```python
from build123d import *

# Parameters (mm, degrees)
SKETCH_1_W          = 120
SKETCH_1_H          = 170
SKETCH_1_R          = 1.7
EXTRUDE_1_DEPTH     = 7
SKETCH_3_R          = 3.4
CUT_EXTRUDE_1_DEPTH = 3
FILLET_1_R          = 5


with BuildPart() as part:
    # 草图1 → 凸台-拉伸1 (new body)
    with BuildSketch(Plane(origin=(0, 0, 0), x_dir=(1, 0, 0), z_dir=(0, 1, 0))):
        with Locations((4.775862069, 0)):
            Rectangle(SKETCH_1_W, SKETCH_1_H)
        with Locations((-8.724137931, 16.5)):
            Circle(SKETCH_1_R, mode=Mode.SUBTRACT)
        with Locations((18.275862069, 16.5)):
            Circle(SKETCH_1_R, mode=Mode.SUBTRACT)
        with Locations((18.275862069, -16.5)):
            Circle(SKETCH_1_R, mode=Mode.SUBTRACT)
        with Locations((-8.724137931, -16.5)):
            Circle(SKETCH_1_R, mode=Mode.SUBTRACT)
        with Locations((-2.724137931, 3)):
            Circle(SKETCH_1_R, mode=Mode.SUBTRACT)
        with Locations((12.275862069, 3)):
            Circle(SKETCH_1_R, mode=Mode.SUBTRACT)
        with BuildLine():
            Line((-15.224137931, 29.7), (24.775862069, 29.7))
            ThreePointArc((24.775862069, 29.7), (27.475862069, 27), (24.775862069, 24.3))
            Line((24.775862069, 24.3), (-15.224137931, 24.3))
            ThreePointArc((-15.224137931, 24.3), (-17.924137931, 27), (-15.224137931, 29.7))
        make_face(mode=Mode.SUBTRACT)
        with BuildLine():
            Line((-15.224137931, 47.3), (24.775862069, 47.3))
            ThreePointArc((24.775862069, 47.3), (27.475862069, 44.6), (24.775862069, 41.9))
            Line((24.775862069, 41.9), (-15.224137931, 41.9))
            ThreePointArc((-15.224137931, 41.9), (-17.924137931, 44.6), (-15.224137931, 47.3))
        make_face(mode=Mode.SUBTRACT)
        with BuildLine():
            Line((-15.224137931, -29.7), (24.775862069, -29.7))
            ThreePointArc((24.775862069, -29.7), (27.475862069, -27), (24.775862069, -24.3))
            Line((24.775862069, -24.3), (-15.224137931, -24.3))
            ThreePointArc((-15.224137931, -24.3), (-17.924137931, -27), (-15.224137931, -29.7))
        make_face(mode=Mode.SUBTRACT)
        with BuildLine():
            Line((-15.224137931, -47.3), (24.775862069, -47.3))
            ThreePointArc((24.775862069, -47.3), (27.475862069, -44.6), (24.775862069, -41.9))
            Line((24.775862069, -41.9), (-15.224137931, -41.9))
            ThreePointArc((-15.224137931, -41.9), (-17.924137931, -44.6), (-15.224137931, -47.3))
        make_face(mode=Mode.SUBTRACT)
        with BuildLine():
            Line((-44.524137931, 44.6), (-44.524137931, -44.6))
            ThreePointArc((-44.524137931, -44.6), (-47.224137931, -47.3), (-49.924137931, -44.6))
            Line((-49.924137931, -44.6), (-49.924137931, 44.6))
            ThreePointArc((-49.924137931, 44.6), (-47.224137931, 47.3), (-44.524137931, 44.6))
        make_face(mode=Mode.SUBTRACT)
        with BuildLine():
            Line((-26.924137931, 44.6), (-26.924137931, -44.6))
            ThreePointArc((-26.924137931, -44.6), (-29.624137931, -47.3), (-32.324137931, -44.6))
            Line((-32.324137931, -44.6), (-32.324137931, 44.6))
            ThreePointArc((-32.324137931, 44.6), (-29.624137931, 47.3), (-26.924137931, 44.6))
        make_face(mode=Mode.SUBTRACT)
        with BuildLine():
            Line((36.475862069, 44.6), (36.475862069, -44.6))
            ThreePointArc((36.475862069, -44.6), (39.175862069, -47.3), (41.875862069, -44.6))
            Line((41.875862069, -44.6), (41.875862069, 44.6))
            ThreePointArc((41.875862069, 44.6), (39.175862069, 47.3), (36.475862069, 44.6))
        make_face(mode=Mode.SUBTRACT)
        with BuildLine():
            Line((54.075862069, 44.6), (54.075862069, -44.6))
            ThreePointArc((54.075862069, -44.6), (56.775862069, -47.3), (59.475862069, -44.6))
            Line((59.475862069, -44.6), (59.475862069, 44.6))
            ThreePointArc((59.475862069, 44.6), (56.775862069, 47.3), (54.075862069, 44.6))
        make_face(mode=Mode.SUBTRACT)
        with BuildLine():
            Line((56.775862069, 56.997520271), (-47.224137931, 56.997520271))
            ThreePointArc((-47.224137931, 56.997520271), (-50.374920197, 60.148302538), (-47.224137931, 63.299084804))
            Line((-47.224137931, 63.299084804), (56.775862069, 63.299084804))
            ThreePointArc((56.775862069, 63.299084804), (59.926644335, 60.148302538), (56.775862069, 56.997520271))
        make_face(mode=Mode.SUBTRACT)
        with BuildLine():
            Line((56.775862069, 70.890661148), (-47.224137931, 70.890661148))
            ThreePointArc((-47.224137931, 70.890661148), (-49.924137931, 73.590661148), (-47.224137931, 76.290661148))
            Line((-47.224137931, 76.290661148), (56.775862069, 76.290661148))
            ThreePointArc((56.775862069, 76.290661148), (59.475862069, 73.590661148), (56.775862069, 70.890661148))
        make_face(mode=Mode.SUBTRACT)
        with BuildLine():
            Line((56.775862069, -56.997520271), (-47.224137931, -56.997520271))
            ThreePointArc((-47.224137931, -56.997520271), (-50.374920197, -60.148302538), (-47.224137931, -63.299084804))
            Line((-47.224137931, -63.299084804), (56.775862069, -63.299084804))
            ThreePointArc((56.775862069, -63.299084804), (59.926644335, -60.148302538), (56.775862069, -56.997520271))
        make_face(mode=Mode.SUBTRACT)
        with BuildLine():
            Line((56.775862069, -70.890661148), (-47.224137931, -70.890661148))
            ThreePointArc((-47.224137931, -70.890661148), (-49.924137931, -73.590661148), (-47.224137931, -76.290661148))
            Line((-47.224137931, -76.290661148), (56.775862069, -76.290661148))
            ThreePointArc((56.775862069, -76.290661148), (59.475862069, -73.590661148), (56.775862069, -70.890661148))
        make_face(mode=Mode.SUBTRACT)
    extrude(amount=EXTRUDE_1_DEPTH)

    # 草图3 → 切除-拉伸1 (cut)
    with BuildSketch(Plane.XZ):
        with Locations((12.275862069, -3)):
            Circle(SKETCH_3_R)
        with Locations((-2.724137931, -3)):
            Circle(SKETCH_3_R)
        with Locations((18.275862069, 16.5)):
            Circle(SKETCH_3_R)
        with Locations((-8.724137931, 16.5)):
            Circle(SKETCH_3_R)
        with Locations((18.275862069, -16.5)):
            Circle(SKETCH_3_R)
        with Locations((-8.724137931, -16.5)):
            Circle(SKETCH_3_R)
    extrude(amount=-CUT_EXTRUDE_1_DEPTH, mode=Mode.SUBTRACT)

    # 圆角1
    fillet_1_edges = [part.edges().sort_by_distance(p)[0] for p in [
        (-55.224137931, 3.5, -85),
        (64.775862069, 3.5, -85),
        (64.775862069, 3.5, 85),
        (-55.224137931, 3.5, 85),
    ]]
    fillet(fillet_1_edges, radius=FILLET_1_R)


solid = part.part
```
Here's how the part is built. I have some questions about the finished solid (model axes, mm). A direction names the side the tool comes from. Round coordinates to 2 decimals unless told otherwise and drop trailing zeros. Order: outer loops, then holes, each group sorted by start corner. A loop starts at its lowest first (then second) coordinate and runs counter-clockwise, first axis right, second up. Notation, with made-up numbers: (-4.75, 24.25) -> (19.25, 24.25) arc R26 ccw to (19.25, 51.25) -> close; hole circle Ø4 at (33, 67). An arc over 180 degrees is marked (long way). Use a Markdown table: item, result. Add a question column.
(1) Suppose I cut it at B-B, the plane z = -11. Please give me the cut outline in (x, y), and give its area (3 significant figures).
(2) For faces 1 (the face through (4, 7, -1)), 2 (the face through (-5.23, 1.48, -0.7)), 3 (the face through (-49.924, 3, 1)), which set-ups out of +Z, -Z, +X, -X, +Y, -Y let a thin tool reach every point of the face, with its end or its side?
(3) If we mould it in two halves opening along Z, with no side actions, what happens to faces 4 (the face through (-47.3, 3.5, -47.3)), 5 (the face through (4, 0, -1)), 6 (the face through (6, 3, -56.998))? For each: released by +Z, released by -Z, zero draft, split by the parting line, or undercut.
(4) Suppose I cut it at C-C, the plane x = 4.5. Count the separate pieces of the cut face and the enclosed holes in it, and give its area (3 significant figures).
(5) Suppose I cut it at A-A, the plane z = 27. Please give me the cut outline in (x, y), and give its area (3 significant figures).
(6) I need wall thicknesses on line 1 along X through (y, z) = (4.75, -36); line 2 along Z through (x, y) = (-18.5, 6.5); line 3 along X through (y, z) = (6, -43.5). Which ranges of each line are inside material? Lowest first, please.
(7) For pin 1 Ø3.5 at (x, z) = (-7.5, 16) entering from -Y, with a flat end and sliding along its axis, tell me the tip position at first contact or that it passes through.
Verdict:
| question | item | result |
|---|---|---|
| 1 | outline | (-55.22, 0) -> (-49.92, 0) -> (-49.92, 7) -> (-55.22, 7) -> close; (-44.52, 0) -> (-32.32, 0) -> (-32.32, 7) -> (-44.52, 7) -> close; (-26.92, 0) -> (36.48, 0) -> (36.48, 7) -> (-26.92, 7) -> close; (41.88, 0) -> (54.08, 0) -> (54.08, 7) -> (41.88, 7) -> close; (59.48, 0) -> (64.78, 0) -> (64.78, 7) -> (59.48, 7) -> close |
| 1 | area | 689 mm2 |
| 2 | face 1 | +Z, -Z, +X, -X, +Y |
| 2 | face 2 | -Y |
| 2 | face 3 | +Y, -Y |
| 3 | face 4 | undercut |
| 3 | face 5 | zero draft |
| 3 | face 6 | undercut |
| 4 | separate pieces | 9 |
| 4 | enclosed holes | 0 |
| 4 | area | 875 mm2 |
| 5 | outline | (-55.22, 0) -> (-49.92, 0) -> (-49.92, 7) -> (-55.22, 7) -> close; (-44.52, 0) -> (-32.32, 0) -> (-32.32, 7) -> (-44.52, 7) -> close; (-26.92, 0) -> (-17.92, 0) -> (-17.92, 7) -> (-26.92, 7) -> close; (27.48, 0) -> (36.48, 0) -> (36.48, 7) -> (27.48, 7) -> close; (41.88, 0) -> (54.08, 0) -> (54.08, 7) -> (41.88, 7) -> close; (59.48, 0) -> (64.78, 0) -> (64.78, 7) -> (59.48, 7) -> close |
| 5 | area | 371 mm2 |
| 6 | line 1 | -55.22 to -49.92, -44.52 to -32.32, -26.92 to 36.48, 41.88 to 54.08, 59.48 to 64.78 |
| 6 | line 2 | -85 to -76.29, -70.89 to -63.3, -57 to 57, 63.3 to 70.89, 76.29 to 85 |
| 6 | line 3 | -55.22 to -49.92, -44.52 to -32.32, -26.92 to -17.69, 27.24 to 36.48, 41.88 to 54.08, 59.48 to 64.78 |
| 7 | pin 1 | y = 3 |
